For this review, take the finished solid that the model builds, in its own axes (mm). Face numbers are marked on the shaded views. A direction names the side the tool comes from. Coordinates: 2 decimals unless noted, no trailing zeros. Write each loop counter-clockwise with the first axis right and the second up, starting at its lowest first coordinate (ties: lowest second). Pieces come first, ordered by that corner, then holes. Notation, with made-up numbers: M 2,8 L 31,8 A27 cw 31,47 Z; hole C 41,-24.75 d5. An arc over 180 degrees is marked long. One line per question, with ' | ' between items.
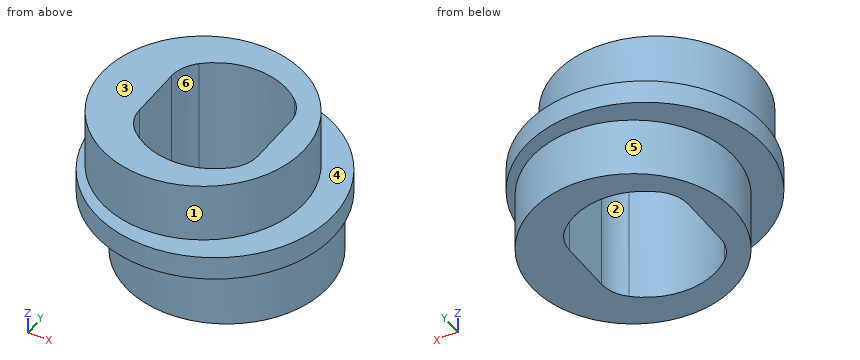
from build123d import *

# Parameters (mm, degrees)
SKETCH1_R           = 8.5
BOSS_EXTRUDE1_DEPTH = 5
SKETCH2_R           = 8.5
BOSS_EXTRUDE2_DEPTH = 7
CUT_EXTRUDE1_DEPTH  = 15.543039572
BOSS_EXTRUDE3_START = 2
SKETCH4_R           = 10
BOSS_EXTRUDE3_DEPTH = 2
FILLET2_R           = 3


with BuildPart() as part:
    # Sketch1 → Boss-Extrude1 (new body)
    with BuildSketch(Plane.XY):
        with Locations((-1, 0)):
            Circle(SKETCH1_R)
        with BuildLine():
            Line((5, -3.31662479), (5, 3.31662479))
            ThreePointArc((5, 3.31662479), (0, 6), (-5, 3.31662479))
            Line((-5, 3.31662479), (-5, -3.31662479))
            ThreePointArc((-5, -3.31662479), (0, -6), (5, -3.31662479))
        make_face(mode=Mode.SUBTRACT)
    extrude(amount=BOSS_EXTRUDE1_DEPTH)

    # Sketch2 → Boss-Extrude2 (add)
    with BuildSketch(Plane(origin=(0, 0, 0), x_dir=(-1, 0, 0), z_dir=(0, 0, -1))):
        with Locations(Location((-1, 0, 0), (0, 0, 276.756327031))):
            Circle(SKETCH2_R)
    extrude(amount=BOSS_EXTRUDE2_DEPTH)

    # Sketch3 → Cut-Extrude1 (cut, through all)
    with BuildSketch(Plane.XY):
        with BuildLine():
            Line((5, -3.31662479), (5, 3.31662479))
            ThreePointArc((5, 3.31662479), (0, 6), (-5, 3.31662479))
            Line((-5, 3.31662479), (-5, -3.31662479))
            ThreePointArc((-5, -3.31662479), (0, -6), (5, -3.31662479))
        make_face()
    extrude(amount=-CUT_EXTRUDE1_DEPTH, mode=Mode.SUBTRACT)

    # Sketch4 → Boss-Extrude3 (add)
    with BuildSketch(Plane(origin=(0, 0, 0), x_dir=(-1, 0, 0), z_dir=(0, 0, -1)).offset(BOSS_EXTRUDE3_START)):
        Circle(SKETCH4_R)
        with BuildLine():
            Line((5, 3.31662479), (5, -3.31662479))
            ThreePointArc((5, -3.31662479), (0, -6), (-5, -3.31662479))
            Line((-5, -3.31662479), (-5, 3.31662479))
            ThreePointArc((-5, 3.31662479), (0, 6), (5, 3.31662479))
        make_face(mode=Mode.SUBTRACT)
    extrude(amount=-BOSS_EXTRUDE3_DEPTH)

    # Fillet2
    fillet2_edges = [part.edges().sort_by_distance(p)[0] for p in [
        (5, 3.31662479, -1),
        (-5, 3.31662479, -1),
        (-5, -3.31662479, -1),
        (5, -3.31662479, -1),
    ]]
    fillet(fillet2_edges, radius=FILLET2_R)


solid = part.part
1. For line 1 along Z through (x, y) = (5.25, 6.5); line 2 along X through (y, z) = (1, -0.5); line 3 along Y through (x, z) = (3.25, -5.25), list the stretches that pass through material, from the lowest coordinate up.
Computed values:
line 1: z = -7 to 0 | line 2: x = -9.95 to -5, 5 to 9.95 | line 3: y = -8.2 to -5.04, 5.04 to 8.2
2. Machinability: for the marked faces 4, 5 and 6, which of the approach directions +Z, -Z, +X, -X, +Y, -Y give a long, thin tool a straight path to every point of the face, cutting with its end or side? Answer none if there is none.
Computed values:
face 4: +Z | face 5: -Z | face 6: +Z, -Z
3. Take a section at D-D on x = 5.5. State the section outline as (y, z) points, plus the area to 3 significant figures.
Computed values:
outline: M -8.35,-2 L -7.21,-2 L -7.21,-7 L 7.21,-7 L 7.21,-2 L 8.35,-2 L 8.35,0 L 5.48,0 L 5.48,5 L -5.48,5 L -5.48,0 L -8.35,0 Z | area: 160 mm2
4. Draft analysis for pull direction Y (two halves, no side actions). For the marked faces 1, 2 and 3, state which applies: pulls with the +Y half, pulls with the -Y half, needs draft (parallel to the pull), parting line crosses it, or undercut.
Computed values:
face 1: parting line crosses it | face 2: undercut | face 3: needs draft
5. Take a section at C-C on z = -3.75. State the section outline as (x, y) points, plus the area to 3 significant figures.
Computed values:
outline: C 1,0 d17; hole M -5,-2.24 A3 ccw -4,-4.47 A6 ccw 4,-4.47 A3 ccw 5,-2.24 L 5,2.24 A3 ccw 4,4.47 A6 ccw -4,4.47 A3 ccw -5,2.24 Z | area: 124 mm2
6. Take a section at A-A on y = 0. State the section outline as (x, z) points.
Computed values:
outline: M -10,-2 L -7.5,-2 L -7.5,-7 L -5,-7 L -5,5 L -9.5,5 L -9.5,0 L -10,0 Z; M 5,-7 L 9.5,-7 L 9.5,-2 L 10,-2 L 10,0 L 7.5,0 L 7.5,5 L 5,5 Z
7. Take a section at B-B on x = 0.5. State the section outline as (y, z) points, plus the area to 3 significant figures.
Computed values:
outline: M -9.99,-2 L -8.49,-2 L -8.49,-7 L -5.98,-7 L -5.98,5 L -8.37,5 L -8.37,0 L -9.99,0 Z; M 5.98,-7 L 8.49,-7 L 8.49,-2 L 9.99,-2 L 9.99,0 L 8.37,0 L 8.37,5 L 5.98,5 Z | area: 65.0 mm2
8. Clearance check with flat-ended pins moving along their axes: P1, Ø1.3, axis at y = 1, z = -2.5, coming from the -X side; P2, Ø3, axis at y = 5.5, z = -2, coming from the +X side; P3, Ø1.5, axis at y = -0.5, z = -3.5, coming from the -X side. State where each tip first meets the part, or that it passes through.
Computed values:
P1: stops at x = -9.98 | P2: stops at x = 9.17 | P3: stops at x = -7.5
